Source: CAD feature listing. Evaluate the final solid. Frame: model axes, mm. A direction names the side the tool comes from. Give positions to 0.01 mm unless a question says otherwise; leave off trailing zeros. Loops run counter-clockwise (first coordinate to the right, second up) from the corner with the lowest first, then second, coordinate; pieces in that order, holes last. Notation, with made-up numbers: (-15, -21) -> (7, -21) arc R22 cw to (7, 3) -> close; hole circle Ø11 at (55.25, 56.25). An arc over 180 degrees is marked (long way). Put each result on its own line as item: value.
Autodesk Inventor part; units mm, degrees
ref_plane "YZ Plane" through (0, 0, 0) normal (1, 0, 0) x (0, 1, 0)
ref_plane "XZ Plane" through (0, 0, 0) normal (0, 1, 0) x (-1, 0, 0)
ref_plane "XY Plane" through (0, 0, 0) normal (0, 0, 1) x (1, 0, 0)
sketch "Sketch1" plane through (0, 0, 0) normal (0, 0, 1) x (1, 0, 0)
  circle A0 centre (0, 0) radius 3
  dimension "d0" = 6
extrude "Extrusion1" add sketch "Sketch1" along normal mid plane 35
sketch "Sketch2" plane through (0, 0, 17.5) normal (0, 0, 1) x (1, 0, 0)
  point P0 (0, 0)
  point P1 (0, 0)
hole "Hole1" at (0, 0, 17.5) direction (0, 0, -1) diameter 2.459 depth 8.8 tip angle 118
sketch "Sketch3" plane through (0, 0, 0) normal (0, 1, 0) x (-1, 0, 0)
  line L0 (3, 2.5) -> (2.5, 2.5)
  line L1 (2.5, 2.5) -> (2.5, 7.5)
  line L2 (2.5, 7.5) -> (3, 7.5)
  line L3 (3, 7.5) -> (3, 2.5)
  line L4 (-3, 7.5) -> (-2.5, 7.5)
  line L5 (-2.5, 7.5) -> (-2.5, 2.5)
  line L6 (-2.5, 2.5) -> (-3, 2.5)
  line L7 (-3, 2.5) -> (-3, 7.5)
  line L8 (-3, -17.5) -> (3, -17.5)
  line L9 (3, 17.5) -> (-3, 17.5)
  point P0 (0, 0)
  point P1 (-3, 23.75)
  dimension "d16" = 0.5
  dimension "d17" = 0.5
  dimension "d18" = 5
  dimension "d19" = 10
extrude "Extrusion2" cut sketch "Sketch3" along normal through all both and the other way through all
mirror "Mirror1" about plane through (0, 0, 0) normal (0, 0, 1) of "Hole1"
equation "\"d17\" = d16"
properties part number "Pancake_Connector" material "Aluminum 6061"
(1) First-contact query: P1, Ø3, axis at y = -1.5, z = 6.5, coming from the -X side; P2, Ø1, axis at y = -0.5, z = 5, coming from the -X side; P3, Ø2, axis at x = 0, y = 0, coming from the +Z side. Flat tips, straight axial feed; report the tip coordinate or a pass-through.
Calculated:
P1: stops at x = -2.98
P2: stops at x = -2.5
P3: stops at z = 8.56
(2) Draft query along X for faces 4 (the flat face through (1, -1, 17.5)), 5 (the flat face through (2.5, 0, 5)), 6 (the conical face through (-0.064, -0.204, -8.09)), 7 (the cylindrical face through (0.748, 0.976, 13.038)). Return one class per face: released by +X, released by -X, zero draft, split by the parting line, or undercut.
Calculated:
face 4: zero draft
face 5: released by +X
face 6: undercut
face 7: undercut
(3) Section A-A on z = 3.5. Return loops of the section in (x, y), then the cut area to 3 significant figures.
Calculated:
outline: (-2.5, -1.66) arc R3 ccw to (2.5, -1.66) -> (2.5, 1.66) arc R3 ccw to (-2.5, 1.66) -> close
area: 26.0 mm²
(4) Section B-B on y = 2.3. Return loops of the section in (x, z), then the cut area to 3 significant figures.
Calculated:
outline: (-1.93, -17.5) -> (1.93, -17.5) -> (1.93, 17.5) -> (-1.93, 17.5) -> close
area: 135 mm²
(5) Line query: probe 1 along X at (y, z) = (0, 11.5); probe 2 along Z at (x, y) = (2.55, -0.5). Output: solid intervals per line, ascending. Write a range as from..to.
Calculated:
probe 1: x = -3..-1.23, 1.23..3
probe 2: z = -17.5..2.5, 7.5..17.5
(6) Reachability of faces 1 (the flat face through (-2.5, 0, 5)), 2 (the conical face through (0.064, -0.204, 8.09)), 3 (the cylindrical face through (-0.748, 0.976, -13.038)) from +Z, -Z, +X, -X, +Y, -Y: full face, straight path, thin tool, end or side. Return the list, or none.
Calculated:
face 1: -X, +Y, -Y
face 2: +Z
face 3: -Z
